```python
from build123d import *

# Parameters (mm, degrees)
SKETCH1_R           = 38.1
SKETCH1_R_2         = 19.05
BOSS_EXTRUDE1_DEPTH = 12.7
SKETCH2_R           = 19.05
BOSS_EXTRUDE3_DEPTH = 69.85
SKETCH3_R           = 12.7
CUT_EXTRUDE1_DEPTH  = 69.85


with BuildPart() as part:
    # Sketch1 → Boss-Extrude1 (new body)
    with BuildSketch(Plane(origin=(0, 0, 0), x_dir=(1, 0, 0), z_dir=(0, 1, 0))):
        with Locations(Location((0, 0, 0), (0, 0, 270))):
            Circle(SKETCH1_R)
        with Locations(Location((0, 0, 0), (0, 0, 270))):
            Circle(SKETCH1_R_2, mode=Mode.SUBTRACT)
    extrude(amount=BOSS_EXTRUDE1_DEPTH)

    # Sketch2 → Boss-Extrude3 (add)
    with BuildSketch(Plane.XZ):
        with Locations(Location((0, 0, 0), (0, 0, 270))):
            Circle(SKETCH2_R)
    extrude(amount=-BOSS_EXTRUDE3_DEPTH)

    # Sketch3 → Cut-Extrude1 (cut)
    with BuildSketch(Plane(origin=(0, 69.85, 0), x_dir=(1, 0, 0), z_dir=(0, 1, 0))):
        with Locations(Location((0, 0, 0), (0, 0, 270))):
            Circle(SKETCH3_R)
    extrude(amount=-CUT_EXTRUDE1_DEPTH, mode=Mode.SUBTRACT)


solid = part.part
```
Can you work these out from the model? Positions are in its coordinate system, mm. A direction names the side the tool comes from. Round coordinates to 2 decimals unless told otherwise and drop trailing zeros. Loops run counter-clockwise (first coordinate to the right, second up) from the corner with the lowest first, then second, coordinate; pieces in that order, holes last.
Item 1: Suppose I cut it at D-D, the plane y = 7. Write out the boundary of the cut face in (x, z).
Item 2: Will these pins go through, and if not, where does the flat tip stop? pin 1 Ø12 at (y, z) = (30.5, -6) entering from -X; pin 2 Ø4 at (y, z) = (37, -12.5) entering from +X; pin 3 Ø5 at (x, z) = (5, -25) entering from +Y.
Item 3: Suppose I cut it at B-B, the plane x = 0. Write out the boundary of the cut face in (y, z), then the cut area to 3 significant figures.
Item 4: Which directions (+Z, -Z, +X, -X, +Y, -Y) give clear straight access to the entire face, cutting with the end or side of a thin tool? Please do faces 4 (the flat face through (-7.9, 12.7, -17.5)), 5 (the flat face through (1, 0, 16)).
Item 5: Please list where these lines run through material, in increasing order: L1, parallel to X at y = 20.5, z = 0; L2, parallel to Y at x = 25, z = 24.5; L3, parallel to Z at x = 4.5, y = 45.
Item 6: If we mould it in two halves opening along X, with no side actions, what happens to faces 1 (the cylindrical face through (-7.7, 35.4, -10.1)), 2 (the cylindrical face through (-11.59, 40.87, 15.12)), 3 (the flat face through (-12.4, 69.85, -4))? For each: +X half, -X half, draft (parallel to the pull), parting line (faces both ways), or undercut.
Item 7: Suppose I cut it at C-C, the plane y = 48.5. Write out the boundary of the cut face in (x, z).
Item 8: Suppose I cut it at A-A, the plane z = 0. Write out the boundary of the cut face in (x, y), then the cut area to 3 significant figures.
Reported:
1. outline: circle Ø76.2 at (0, 0); hole circle Ø25.4 at (0, 0)
2. pin 1: stops at x = -19.05
2. pin 2: stops at x = 15.9
2. pin 3: stops at y = 12.7
3. outline: (0, -38.1) - (12.7, -38.1) - (12.7, -19.05) - (69.85, -19.05) - (69.85, -12.7) - (0, -12.7) - close; (0, 12.7) - (69.85, 12.7) - (69.85, 19.05) - (12.7, 19.05) - (12.7, 38.1) - (0, 38.1) - close
3. area: 1,370 mm2
4. face 4: +Y
4. face 5: +Z, -Z, +X, -X, -Y
5. L1: x = -19.05 to -12.7, 12.7 to 19.05
5. L2: y = 0 to 12.7
5. L3: z = -18.51 to -11.88, 11.88 to 18.51
6. face 1: undercut
6. face 2: parting line
6. face 3: draft
7. outline: circle Ø38.1 at (0, 0); hole circle Ø25.4 at (0, 0)
8. outline: (-38.1, 0) - (-12.7, 0) - (-12.7, 69.85) - (-19.05, 69.85) - (-19.05, 12.7) - (-38.1, 12.7) - close; (12.7, 0) - (38.1, 0) - (38.1, 12.7) - (19.05, 12.7) - (19.05, 69.85) - (12.7, 69.85) - close
8. area: 1,370 mm2
